```python
from build123d import *

# Parameters (mm, degrees)
BASE_FLANGE1_START             = -2
BASE_FLANGE1_OUTLINE_R         = 2.25
BASE_FLANGE1_OUTLINE_R_2       = 9.75
BASE_FLANGE1_DEPTH             = 2
EDGE_FLANGE1_STRIP_W           = 9.4732
EDGE_FLANGE1_STRIP_H           = 2
EDGE_FLANGE1_STRIP_CUT_DEPTH   = 220
EDGE_FLANGE1_STRIP_2_W         = 9.4732
EDGE_FLANGE1_STRIP_2_H         = 2
EDGE_FLANGE1_STRIP_CUT_2_DEPTH = 220
EDGE_FLANGE1_DEPTH             = 220
EDGE_FLANGE1_BEND_DEPTH        = 220
EDGE_FLANGE2_STRIP_W           = 9.4732
EDGE_FLANGE2_STRIP_H           = 2
EDGE_FLANGE2_STRIP_CUT_DEPTH   = 43
EDGE_FLANGE2_STRIP_2_W         = 9.4732
EDGE_FLANGE2_STRIP_2_H         = 2
EDGE_FLANGE2_STRIP_CUT_2_DEPTH = 43
EDGE_FLANGE2_DEPTH             = 43
EDGE_FLANGE2_BEND_DEPTH        = 43
SKETCH19_R                     = 2
CUT_EXTRUDE3_DEPTH             = 229.228503917
CUT_EXTRUDE4_DEPTH             = 121.814941129


# Read off the part's stored shape, not the designer's step: Base-Flange1
# Sheet-metal steps are written as plain solids
with BuildPart() as part:
    # Base-Flange1 outline → Base-Flange1 (new body)
    with BuildSketch(Plane(origin=(0, 0, 0), x_dir=(1, 0, 0), z_dir=(0, 1, 0)).offset(BASE_FLANGE1_START)):
        Polygon((108, 23.5), (110, 23.5), (110, 27.5), (-110, 27.5), (-110, 23.5), (-108, 23.5), (-108, 21.5), (-110, 21.5), (-110, -21.5), (-108, -21.5), (-108, -23.5), (-110, -23.5), (-110, -27.5), (110, -27.5), (110, -23.5), (108, -23.5), (108, -21.5), (110, -21.5), (110, 21.5), (108, 21.5), align=None)
        with Locations((-67.5, -10)):
            Circle(BASE_FLANGE1_OUTLINE_R, mode=Mode.SUBTRACT)
        with BuildLine():
            ThreePointArc((-25, -21.75), (-40.25, -6.5), (-25, 8.75))
            Line((-25, 8.75), (25, 8.75))
            ThreePointArc((25, 8.75), (40.25, -6.5), (25, -21.75))
            Line((25, -21.75), (-25, -21.75))
        make_face(mode=Mode.SUBTRACT)
        with Locations((67.5, -10)):
            Circle(BASE_FLANGE1_OUTLINE_R, mode=Mode.SUBTRACT)
        with Locations((-82, 4.5)):
            Circle(BASE_FLANGE1_OUTLINE_R, mode=Mode.SUBTRACT)
        with Locations((-67.5, 4.5)):
            Circle(BASE_FLANGE1_OUTLINE_R_2, mode=Mode.SUBTRACT)
        with Locations((-53, 4.5)):
            Circle(BASE_FLANGE1_OUTLINE_R, mode=Mode.SUBTRACT)
        with Locations((-67.5, 19)):
            Circle(BASE_FLANGE1_OUTLINE_R, mode=Mode.SUBTRACT)
        with Locations((53, 4.5)):
            Circle(BASE_FLANGE1_OUTLINE_R, mode=Mode.SUBTRACT)
        with Locations((67.5, 4.5)):
            Circle(BASE_FLANGE1_OUTLINE_R_2, mode=Mode.SUBTRACT)
        with Locations((82, 4.5)):
            Circle(BASE_FLANGE1_OUTLINE_R, mode=Mode.SUBTRACT)
        with Locations((67.5, 19)):
            Circle(BASE_FLANGE1_OUTLINE_R, mode=Mode.SUBTRACT)
    extrude(amount=BASE_FLANGE1_DEPTH)

    # Edge-Flange1 strip (across the edge) → Edge-Flange1 strip cut (cut)
    with BuildSketch(Plane(origin=(110, 0, -27.5), x_dir=(0, 0, 1), z_dir=(-1, 0, 0))):
        with Locations((-2, -1)):
            Rectangle(EDGE_FLANGE1_STRIP_W, EDGE_FLANGE1_STRIP_H)
    extrude(amount=EDGE_FLANGE1_STRIP_CUT_DEPTH, mode=Mode.SUBTRACT)

    # Edge-Flange1 strip 2 (across the edge) → Edge-Flange1 strip cut 2 (cut)
    with BuildSketch(Plane(origin=(-110, 0, 27.5), x_dir=(0, 0, -1), z_dir=(1, 0, 0))):
        with Locations((-2, -1)):
            Rectangle(EDGE_FLANGE1_STRIP_2_W, EDGE_FLANGE1_STRIP_2_H)
    extrude(amount=EDGE_FLANGE1_STRIP_CUT_2_DEPTH, mode=Mode.SUBTRACT)

    # Edge-Flange1 section (across the edge) → Edge-Flange1 (add)
    with BuildSketch(Plane(origin=(110, 0, -27.5), x_dir=(0, 0, 1), z_dir=(-1, 0, 0))):
        with BuildLine():
            Line((0, 0.7366), (0, 2))
            Line((0, 2), (2, 2))
            Line((2, 2), (2, 0.7366))
            ThreePointArc((2, 0.7366), (2.215745145, 0.215745145), (2.7366, 0))
            Line((2.7366, 0), (2.7366, -2))
            ThreePointArc((2.7366, -2), (0.801531583, -1.198468417), (0, 0.7366))
        make_face()
    extrude(amount=EDGE_FLANGE1_DEPTH)

    # Edge-Flange1 section 2 (across the edge) → Edge-Flange1 bend (add)
    with BuildSketch(Plane(origin=(-110, 0, 27.5), x_dir=(0, 0, -1), z_dir=(1, 0, 0))):
        with BuildLine():
            Line((0, 0.7366), (0, 2))
            Line((0, 2), (2, 2))
            Line((2, 2), (2, 0.7366))
            ThreePointArc((2, 0.7366), (2.215745145, 0.215745145), (2.7366, 0))
            Line((2.7366, 0), (2.7366, -2))
            ThreePointArc((2.7366, -2), (0.801531583, -1.198468417), (0, 0.7366))
        make_face()
    extrude(amount=EDGE_FLANGE1_BEND_DEPTH)

    # Edge-Flange2 strip (across the edge) → Edge-Flange2 strip cut (cut)
    with BuildSketch(Plane(origin=(-110, 0, -21.5), x_dir=(1, 0, 0), z_dir=(0, 0, 1))):
        with Locations((-4, -1)):
            Rectangle(EDGE_FLANGE2_STRIP_W, EDGE_FLANGE2_STRIP_H)
    extrude(amount=EDGE_FLANGE2_STRIP_CUT_DEPTH, mode=Mode.SUBTRACT)

    # Edge-Flange2 strip 2 (across the edge) → Edge-Flange2 strip cut 2 (cut)
    with BuildSketch(Plane(origin=(110, 0, 21.5), x_dir=(-1, 0, 0), z_dir=(0, 0, -1))):
        with Locations((-4, -1)):
            Rectangle(EDGE_FLANGE2_STRIP_2_W, EDGE_FLANGE2_STRIP_2_H)
    extrude(amount=EDGE_FLANGE2_STRIP_CUT_2_DEPTH, mode=Mode.SUBTRACT)

    # Edge-Flange2 section (across the edge) → Edge-Flange2 (add)
    with BuildSketch(Plane(origin=(-110, 0, -21.5), x_dir=(1, 0, 0), z_dir=(0, 0, 1))):
        with BuildLine():
            Line((-2, 0.7366), (-2, 34))
            Line((-2, 34), (0, 34))
            Line((0, 34), (0, 0.7366))
            ThreePointArc((0, 0.7366), (0.215745145, 0.215745145), (0.7366, 0))
            Line((0.7366, 0), (0.7366, -2))
            ThreePointArc((0.7366, -2), (-1.198468417, -1.198468417), (-2, 0.7366))
        make_face()
    extrude(amount=EDGE_FLANGE2_DEPTH)

    # Edge-Flange2 section 2 (across the edge) → Edge-Flange2 bend (add)
    with BuildSketch(Plane(origin=(110, 0, 21.5), x_dir=(-1, 0, 0), z_dir=(0, 0, -1))):
        with BuildLine():
            Line((-2, 0.7366), (-2, 34))
            Line((-2, 34), (0, 34))
            Line((0, 34), (0, 0.7366))
            ThreePointArc((0, 0.7366), (0.215745145, 0.215745145), (0.7366, 0))
            Line((0.7366, 0), (0.7366, -2))
            ThreePointArc((0.7366, -2), (-1.198468417, -1.198468417), (-2, 0.7366))
        make_face()
    extrude(amount=EDGE_FLANGE2_BEND_DEPTH)

    # Sketch19 → Cut-Extrude3 (cut, through all)
    with BuildSketch(Plane.ZY.offset(112)):
        with Locations(Location((-16.5, 28, 0), (0, 0, 270))):
            Circle(SKETCH19_R)
        with Locations(Location((-16.5, 8, 0), (0, 0, 270))):
            Circle(SKETCH19_R)
        with Locations(Location((16.5, 8, 0), (0, 0, 270))):
            Circle(SKETCH19_R)
        with Locations(Location((16.5, 28, 0), (0, 0, 270))):
            Circle(SKETCH19_R)
    extrude(amount=-CUT_EXTRUDE3_DEPTH, mode=Mode.SUBTRACT)

    # Sketch22 → Cut-Extrude4 (cut, through all)
    with BuildSketch(Plane.XZ.offset(2)):
        Polygon((-108, 23.5), (-110, 23.5), (-110, 24.7634), (-110, 27.5), (-108, 27.5), align=None)
        Polygon((-108, -23.5), (-108, -27.5), (-110, -27.5), (-110, -24.7634), (-110, -23.5), align=None)
        Polygon((108, -23.5), (110, -23.5), (110, -24.7634), (110, -27.5), (108, -27.5), align=None)
        Polygon((108, 23.5), (108, 27.5), (110, 27.5), (110, 24.7634), (110, 23.5), align=None)
    extrude(amount=-CUT_EXTRUDE4_DEPTH, mode=Mode.SUBTRACT)


solid = part.part
```
Input: part model. Units: mm. Frame: model coordinates. A direction names the side the tool comes from. Coordinates: 2 decimals unless noted, no trailing zeros. Write each loop counter-clockwise with the first axis right and the second up, starting at its lowest first coordinate (ties: lowest second). Pieces come first, ordered by that corner, then holes. Notation, with made-up numbers: (75, 39) -> (122, 39) arc R25 ccw to (122, 63) -> close; hole circle Ø10 at (67.5, 36). An arc over 180 degrees is marked (long way). Answer as a JSON object with one key per item and string values.
1. First-contact query: P1, Ø7, axis at x = 67.5, z = -19, coming from the +Y side; P2, Ø0.6, axis at x = 4.5, y = -0.5, coming from the -Z side; P3, Ø2, axis at y = -1, z = 26, coming from the -X side. Flat tips, straight axial feed; report the tip coordinate or a pass-through.
Result set:
{"P1": "stops at y = 0", "P2": "stops at z = -27.33", "P3": "stops at x = -108"}
2. Section B-B on x = -53. Return the cut outline in (y, z), then the cut area to 3 significant figures.
Result set:
{"outline": "(-2, -24.76) arc R2.74 ccw to (0.74, -27.5) -> (2, -27.5) -> (2, -25.5) -> (0.74, -25.5) arc R0.74 cw to (0, -24.76) -> (0, -6.75) -> (-2, -6.75) -> close; (-2, -2.25) -> (0, -2.25) -> (0, 24.76) arc R0.74 cw to (0.74, 25.5) -> (2, 25.5) -> (2, 27.5) -> (0.74, 27.5) arc R2.74 ccw to (-2, 24.76) -> close", "area": "106 mm2"}
3. Section C-C on z = 10. Return the cut outline in (x, y).
Result set:
{"outline": "(-112, 0.74) arc R2.74 ccw to (-109.26, -2) -> (-69.75, -2) -> (-69.75, 0) -> (-109.26, 0) arc R0.74 cw to (-110, 0.74) -> (-110, 34) -> (-112, 34) -> close; (-65.25, -2) -> (-39.84, -2) -> (-39.84, 0) -> (-65.25, 0) -> close; (39.84, -2) -> (65.25, -2) -> (65.25, 0) -> (39.84, 0) -> close; (69.75, -2) -> (109.26, -2) arc R2.74 ccw to (112, 0.74) -> (112, 34) -> (110, 34) -> (110, 0.74) arc R0.74 cw to (109.26, 0) -> (69.75, 0) -> close"}
4. Material intervals for line 1 (X direction, y = 5, z = 20.5); line 2 (Z direction, x = 110.7, y = 8); line 3 (X direction, y = -1.45, z = 10), sorted ascending. Write a range as from..to.
Result set:
{"line 1": "x = -112..-110, 110..112", "line 2": "z = -21.5..-18.5, -14.5..14.5, 18.5..21.5", "line 3": "x = -110.91..-69.75, -65.25..-39.84, 39.84..65.25, 69.75..110.91"}
5. Mould query, pull axis X, two halves, no side actions, for faces 5 (the face through (112, 17, 0)), 6 (the face through (-111.014, 8.26, 18.483)), 7 (the face through (65.84, -1.01, 8.48)), 8 (the face through (84.08, -1.01, -3.64)). Classes: released by +X, released by -X, zero draft, split by the parting line, or undercut.
Result set:
{"face 5": "released by +X", "face 6": "zero draft", "face 7": "undercut", "face 8": "undercut"}
6. Section A-A on y = 13.5. Return the cut outline in (x, z).
Result set:
{"outline": "(-112, -21.5) -> (-110, -21.5) -> (-110, 21.5) -> (-112, 21.5) -> close; (110, -21.5) -> (112, -21.5) -> (112, 21.5) -> (110, 21.5) -> close"}
7. Section D-D on z = -4.5. Count the separate pieces of the cut face and the enclosed holes in it, then the cut area to 3 significant figures.
Result set:
{"separate pieces": "8", "enclosed holes": "0", "area": "325 mm2"}
8. Access query for faces 1 (the face through (110, 18, 0)), 2 (the face through (108, -0.5, -24.5)), 3 (the face through (-108, -0.5, -24.5)), 4 (the face through (40.246, -1.014, 6.165)). Directions: +Z, -Z, +X, -X, +Y, -Y. A direction counts if a zero-diameter tool reaches every point of the face in a straight line with its end or side. Return the directions, or none.
Result set:
{"face 1": "+Z, -Z, +Y", "face 2": "-Z, +X, +Y, -Y", "face 3": "-Z, -X, +Y, -Y", "face 4": "+Y, -Y"}
